Solid Edge part; units mm, degrees
sketch "Sketch1" plane through (0, 0, 0) normal (0, 0, 1) x (1, 0, 0)
  circle A0 centre (0, 0) radius 1.621
  circle A1 centre (0, 0) radius 4.0415
extrude "Protrusion1" add sketch "Sketch1" along normal blind 2.2
sketch "Sketch2" plane through (0, 0, 0) normal (0, 0, 1) x (1, 0, 0)
  line L0 (4.0415, 0) -> (2.0207, 3.5)
  arc A0 (2.0207, 3.5) -> (4.0415, 0) centre (0, 0) cw
extrude "ExtrudedCutout_1" cut sketch "Sketch2" along normal blind 2.2
pattern_circular "Pattern1" count 6 over 360 about axis through (0, 0, 0) along (0, 0, -1) of "ExtrudedCutout_1"
cosmetic_thread "Thread_1" thread depth 2.2
sketch "Sketch3" plane through (0, 0, 0) normal (0, -1, 0) x (1, 0, 0)
  line L0 (4.0415, 0.1484) -> (3.4875, 0)
  line L1 (3.4875, 0) -> (4.0415, 0)
  line L2 (4.0415, 0) -> (4.0415, 0.1484)
  line L3 (3.4875, 2.2) -> (4.0415, 2.2)
  line L4 (4.0415, 2.2) -> (4.0415, 2.0516)
  line L5 (4.0415, 2.0516) -> (3.4875, 2.2)
revolve "RevolvedCutout_1" cut sketch "Sketch3" angle 360 about axis through (0, 0, 8.4) along (0, 0, -1)
chamfer "Chamfer_1" distance 0.679 angle 30 1 edges at (-1.621, 0, 0) measured on face at (-2.3947, -2.2552, 0)
chamfer "Chamfer_2" distance 0.679 angle 30 1 edges at (-1.621, 0, 2.2) measured on face at (-2.3947, -2.2552, 2.2)
properties material "Steel"
Geometry check sheet. Reference: the model listing, model coordinates, mm. Give positions to 0.01 mm unless a question says otherwise; leave off trailing zeros. Loops run counter-clockwise (first coordinate to the right, second up) from the corner with the lowest first, then second, coordinate; pieces in that order, holes last. Notation, with made-up numbers: (-15, 76) - (12, 76) arc R33 ccw to (12, 113) - close; hole circle Ø5 at (52.5, 31). An arc over 180 degrees is marked (long way). Use CSV: the item, a comma, the result in double quotes. Start each with the question number.
Q1. Release check for a two-part mould opening along Y. For faces 1 (the face through (3, -1.8, 1.1)), 2 (the face through (3.045, 1.726, 1.085)), 3 (the face through (0.748, 1.438, 1.09)) record: +Y half, -Y half, draft (parallel to the pull), parting line (faces both ways), or undercut.
Q2. Section check B-B, the plane z = 1.2. Record the cut outline in (x, y), and give its area (3 significant figures).
Q3. Scan lines: probe 1 along Y at (x, z) = (0, 0.9); probe 2 along X at (y, z) = (-1.25, 0.2); probe 3 along X at (y, z) = (-0.5, 1.2). Record each from-to range of solid material in increasing order. Write a range as from..to.
Findings below:
1,face 1,"-Y half"
1,face 2,"+Y half"
1,face 3,"undercut"
2,outline,"(-4.04, 0) - (-2.02, -3.5) - (2.02, -3.5) - (4.04, 0) - (2.02, 3.5) - (-2.02, 3.5) - close; hole circle Ø3.24 at (0, 0)"
2,area,"34.2 mm^2"
3,probe 1,"y = -3.5..-1.62, 1.62..3.5"
3,probe 2,"x = -3.32..-1.5, 1.5..3.32"
3,probe 3,"x = -3.75..-1.54, 1.54..3.75"
